The model under review builds one solid part; all positions refer to its coordinate system, in mm. A direction names the side the tool comes from. Coordinates: 2 decimals unless noted, no trailing zeros. Order: outer loops, then holes, each group sorted by start corner. A loop starts at its lowest first (then second) coordinate and runs counter-clockwise, first axis right, second up. Notation, with made-up numbers: M -32,14.5 L 5,14.5 A18 ccw 5,31.5 Z; hole C -7,-25.75 d8. An arc over 180 degrees is marked long. Answer as CSV lines item,"result". Start each with the question number.
Q1. The part is to be moulded in two halves that separate along X. For faces 4 (the face through (-14.8, 1.9, 0)), 5 (the face through (21, 3, 4)), 6 (the face through (-16.234, 1.715, 4.056)), say which applies: +X half, -X half, draft (parallel to the pull), parting line (faces both ways), or undercut.
Q2. Wall thickness on L1, parallel to Y at x = -16, z = 4; L2, parallel to X at y = 2.5, z = 2.75; L3, parallel to X at y = 2, z = 3.5: over which ranges is each line inside the solid? List them lowest first. Write a range as [from, to].
Q3. Machinability: for faces 1 (the face through (-18, 3, 8)), 2 (the face through (18, 3, 8)), 3 (the face through (0, 7, 12)), which of the approach directions +Z, -Z, +X, -X, +Y, -Y give a long, thin tool a straight path to every point of the face, cutting with its end or side? Answer none if there is none.
Q4. Consider section B-B on x = 16. Write out the cut boundary in (y, z).
Q5. Consider section C-C on y = 3.5. Write out the cut boundary in (x, z).
Q6. Consider section D-D on x = 0. Write out the cut boundary in (y, z).
Q7. For P1, Ø3.5, axis at x = 17.5, y = 4.5, coming from the +Z side; P2, Ø4, axis at y = 2, z = 12.5, coming from the -X side; P3, Ø4, axis at x = -16, y = 3.5, coming from the -Z side; P4, Ø1, axis at x = 0, y = 3, coming from the -Z side, all flat-tipped, find the tip position at first contact; note any pin that passes through.
Q8. Consider section A-A on z = 2.5. Write out the cut boundary in (x, y), and give its area (3 significant figures).
from build123d import *

# Parameters (mm, degrees)
BOSS_EXTRUDE1_DEPTH = 7
SKETCH4_R           = 1.8
CUT_EXTRUDE3_DEPTH  = 27.739483914


with BuildPart() as part:
    # Sketch3 → Boss-Extrude1 (new body)
    with BuildSketch(Plane(origin=(0, 0, 0), x_dir=(1, 0, 0), z_dir=(0, 1, 0))):
        with BuildLine():
            Line((-11, 0), (-21, 0))
            Line((-21, 0), (-21, -8))
            Line((-21, -8), (-12.68857754, -8))
            ThreePointArc((-12.68857754, -8), (0, -15), (12.68857754, -8))
            Line((12.68857754, -8), (21, -8))
            Line((21, -8), (21, 0))
            Line((21, 0), (11, 0))
            ThreePointArc((11, 0), (0, -11), (-11, 0))
        make_face()
    extrude(amount=BOSS_EXTRUDE1_DEPTH)

    # Sketch4 → Cut-Extrude3 (cut, symmetric)
    with BuildSketch(Plane.XY):
        with Locations(Location((16, 3.5, 0), (0, 0, 180))):
            Circle(SKETCH4_R)
    cut_extrude3 = extrude(amount=CUT_EXTRUDE3_DEPTH, both=True, mode=Mode.SUBTRACT)

    # Mirror1: Cut-Extrude3 across plane
    add(cut_extrude3.mirror(Plane(origin=(0, 0, 0), x_dir=(0, 0, 1), z_dir=(1, 0, 0))), mode=Mode.SUBTRACT)


solid = part.part
Evaluation:
1,face 4,"draft"
1,face 5,"+X half"
1,face 6,"undercut"
2,L1,"y = [0, 1.7], [5.3, 7]"
2,L2,"x = [-21, -17.5], [-14.5, -10.65], [10.65, 14.5], [17.5, 21]"
2,L3,"x = [-21, -16.99], [-15.01, -10.43], [10.43, 15.01], [16.99, 21]"
3,face 1,"+Z, -X, +Y, -Y"
3,face 2,"+Z, +X, +Y, -Y"
3,face 3,"+Z, -Z, +X, -X, +Y"
4,outline,"M 0,0 L 1.7,0 L 1.7,8 L 0,8 Z; M 5.3,0 L 7,0 L 7,8 L 5.3,8 Z"
5,outline,"M -21,0 L -17.8,0 L -17.8,8 L -21,8 Z; M -14.2,0 L -11,0 A11 cw 11,0 L 14.2,0 L 14.2,8 L 12.69,8 A15 ccw -12.69,8 L -14.2,8 Z; M 17.8,0 L 21,0 L 21,8 L 17.8,8 Z"
6,outline,"M 0,11 L 7,11 L 7,15 L 0,15 Z"
7,P1,"stops at z = 8"
7,P2,"stops at x = -10.71"
7,P3,"stops at z = 0"
7,P4,"stops at z = 10.99"
8,outline,"M -21,0 L -10.71,0 L -10.71,7 L -21,7 Z; M 10.71,0 L 21,0 L 21,7 L 10.71,7 Z; hole C -16,3.5 d3.6; hole C 16,3.5 d3.6"
8,area,"124 mm²"
